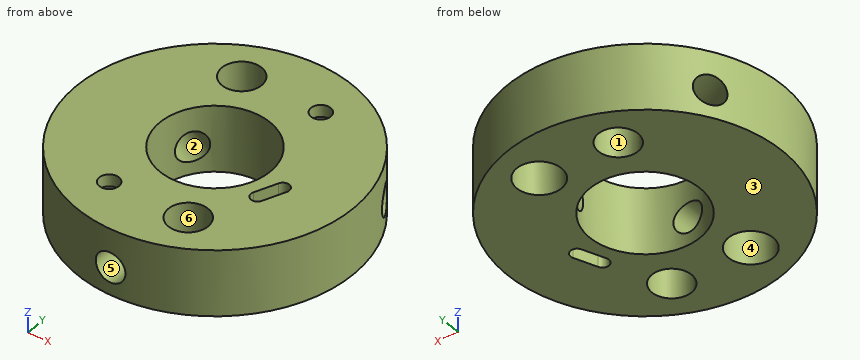
from build123d import *

# Parameters (mm, degrees)
SKETCH1_R                                      = 15.875
BOSS_EXTRUDE1_DEPTH                            = 7.62
SKETCH2_R                                      = 6.35
CUT_EXTRUDE1_DEPTH                             = 24.708556472
CIRPATTERN1_COUNT                              = 3
CBORE_FOR_2_BUTTON_HEAD_CAP_SCREW1_D           = 2.2606
CBORE_FOR_2_BUTTON_HEAD_CAP_SCREW1_CBORE_D     = 5.15874
CBORE_FOR_2_BUTTON_HEAD_CAP_SCREW1_CBORE_DEPTH = 6.2484
CIRPATTERN2_COUNT                              = 2
SKETCH42_R                                     = 2.286
CUT_EXTRUDE2_DEPTH                             = 7.62
CIRPATTERN3_COUNT                              = 2
CUT_EXTRUDE3_DEPTH                             = 24.70855664


with BuildPart() as part:
    # Sketch1 → Boss-Extrude1 (new body)
    with BuildSketch(Plane.XY):
        with Locations(Location((0, 0, 0), (0, 0, 180))):
            Circle(SKETCH1_R)
    extrude(amount=BOSS_EXTRUDE1_DEPTH)

    # Sketch2 → Cut-Extrude1 (cut, through all)
    with BuildSketch(Plane.XY.offset(7.62)):
        Circle(SKETCH2_R)
    extrude(amount=-CUT_EXTRUDE1_DEPTH, mode=Mode.SUBTRACT)

    # Sketch36 → Tap Drill for #8-32 Tap1 (revolve, cut)
    with BuildSketch(Plane(origin=(-0.450397279, -15.875, 3.175), x_dir=(0, 0, -1), z_dir=(1, 0, 0))):
        Polygon((0, 0), (0, 20.499292883), (1.7272, 19.05), (1.7272, 0), align=None)
    tap_drill_for_8_32_tap1 = revolve(axis=Axis((-0.450397279, -22.225, 3.175), (0, 1, 0)), mode=Mode.SUBTRACT)

    # CirPattern1: Tap Drill for #8-32 Tap1 ×3 about axis
    cirpattern1_axis = Axis((0, 0, 7.62), (0, 0, -1))
    for i in range(1, CIRPATTERN1_COUNT):
        add(tap_drill_for_8_32_tap1.rotate(cirpattern1_axis, i * 360 / CIRPATTERN1_COUNT), mode=Mode.SUBTRACT)

    # CBORE for #2 Button Head Cap Screw1 (through all)
    with Locations(Plane(origin=(0, 0, 0), x_dir=(-1, 0, 0), z_dir=(0, 0, -1))):
        with Locations((4.769587089, -10.050926029)):
            cbore_for_2_button_head_cap_screw1 = CounterBoreHole(CBORE_FOR_2_BUTTON_HEAD_CAP_SCREW1_D / 2, CBORE_FOR_2_BUTTON_HEAD_CAP_SCREW1_CBORE_D / 2, CBORE_FOR_2_BUTTON_HEAD_CAP_SCREW1_CBORE_DEPTH)

    # CirPattern2: CBORE for #2 Button Head Cap Screw1 ×2 about axis
    cirpattern2_axis = Axis((0, 0, 0), (0, 0, 1))
    for i in range(1, CIRPATTERN2_COUNT):
        add(cbore_for_2_button_head_cap_screw1.rotate(cirpattern2_axis, i * 360 / CIRPATTERN2_COUNT), mode=Mode.SUBTRACT)

    # Sketch42 → Cut-Extrude2 (cut)
    with BuildSketch(Plane(origin=(0, 0, 0), x_dir=(-1, 0, 0), z_dir=(0, 0, -1))):
        with Locations((4.365368762, 10.219159056)):
            Circle(SKETCH42_R)
    cut_extrude2 = extrude(amount=-CUT_EXTRUDE2_DEPTH, mode=Mode.SUBTRACT)

    # CirPattern3: Cut-Extrude2 ×2 about axis
    cirpattern3_axis = Axis((0, 0, 0), (0, 0, 1))
    for i in range(1, CIRPATTERN3_COUNT):
        add(cut_extrude2.rotate(cirpattern3_axis, i * 360 / CIRPATTERN3_COUNT), mode=Mode.SUBTRACT)

    # Sketch43 → Cut-Extrude3 (cut, through all)
    with BuildSketch(Plane(origin=(0, 0, 0), x_dir=(-1, 0, 0), z_dir=(0, 0, -1))):
        with BuildLine():
            Line((-8.025711128, -1.073137194), (-6.956985206, -3.563699487))
            ThreePointArc((-6.956985206, -3.563699487), (-7.355887027, -4.562271884), (-8.354459424, -4.163370063))
            Line((-8.354459424, -4.163370063), (-9.423185347, -1.67280777))
            ThreePointArc((-9.423185347, -1.67280777), (-9.024283525, -0.674235373), (-8.025711128, -1.073137194))
        make_face()
    extrude(amount=-CUT_EXTRUDE3_DEPTH, mode=Mode.SUBTRACT)


solid = part.part
Can you work these out from the model? Positions are in its coordinate system, mm. Face numbers are marked on the shaded views. A direction names the side the tool comes from. Give positions to 0.01 mm unless a question says otherwise; leave off trailing zeros. Loops run counter-clockwise (first coordinate to the right, second up) from the corner with the lowest first, then second, coordinate; pieces in that order, holes last. Notation, with made-up numbers: (51, 85.5) -> (79, 85.5) arc R30 cw to (79, 112.5) -> close; hole circle Ø8 at (-28, -33). An arc over 180 degrees is marked (long way). Return JSON: item names as keys, results as strings.
Q1. I want a section at A-A, the plane z = 2.5. List the corners of the cut face in (x, y) for me (3 decimals).
Checks:
{"outline": "(-14.282, 6.93) arc R15.875 ccw to (-2.04, -15.743) -> (-2.04, -6.013) arc R6.35 cw to (-5.98, 2.137) -> close; (-12.614, 9.639) -> (-4.188, 4.774) arc R6.35 cw to (4.84, 4.11) -> (13.143, 8.904) arc R15.875 ccw to start; (1.139, -15.834) arc R15.875 ccw to (14.654, 6.105) -> (6.228, 1.24) arc R6.35 cw to (1.139, -6.247) -> close; hole circle Ø5.159 at (-4.77, -10.051); hole circle Ø4.572 at (-4.365, 10.219); hole circle Ø4.572 at (4.365, -10.219); hole circle Ø5.159 at (4.77, 10.051); hole (6.957, -3.564) arc R0.76 ccw to (8.354, -4.163) -> (9.423, -1.673) arc R0.76 ccw to (8.026, -1.073) -> close"}
Q2. We'd pull the mould along Z, two halves only. Please class the marked faces 1, 2 and 3: released by +Z, released by -Z, zero draft, split by the parting line, or undercut.
Checks:
{"face 1": "zero draft", "face 2": "undercut", "face 3": "released by -Z"}
Q3. On a 3-axis mill with a long thin cutter (end or side, diameter ignored), from which of +Z, -Z, +X, -X, +Y, -Y can I reach the whole of each face in a straight line? I mean the marked faces 4, 5 and 6. Say none if no direction works.
Checks:
{"face 4": "-Z", "face 5": "-Y", "face 6": "+Z, -Z"}
Q4. I want a section at D-D, the plane z = 7. List the corners of the cut face in (x, y) for me (3 decimals), then the cut area to 3 significant figures.
Checks:
{"outline": "circle Ø31.75 at (0, 0); hole circle Ø4.572 at (-4.365, 10.219); hole circle Ø12.7 at (0, 0); hole circle Ø2.261 at (-4.77, -10.051); hole circle Ø4.572 at (4.365, -10.219); hole circle Ø2.261 at (4.77, 10.051); hole (6.957, -3.564) arc R0.76 ccw to (8.354, -4.163) -> (9.423, -1.673) arc R0.76 ccw to (8.026, -1.073) -> close", "area": "618 mm2"}
Q5. I want a section at C-C, the plane x = 3. List the corners of the cut face in (y, z) for me, then the cut area to 3 significant figures.
Checks:
{"outline": "(-15.59, 0) -> (-12.05, 0) -> (-12.05, 7.62) -> (-15.59, 7.62) -> close; (-8.39, 0) -> (-5.6, 0) -> (-5.6, 7.62) -> (-8.39, 7.62) -> close; (5.6, 0) -> (8.17, 0) -> (8.17, 6.25) -> (11.93, 6.25) -> (11.93, 0) -> (15.59, 0) -> (15.59, 7.62) -> (5.6, 7.62) -> close", "area": "101 mm2"}
Q6. For pin 1 Ø4 at (x, y) = (-4.5, -9) entering from -Z; pin 2 Ø1.5 at (y, z) = (8, 2) entering from -X; pin 3 Ø1.5 at (x, y) = (6, 11) entering from -Z; pin 4 Ø3 at (x, z) = (4, 4.5) entering from -Y, each with a flat end and sliding along its axis, tell me the tip position at first contact or that it passes through.
Checks:
{"pin 1": "stops at z = 0", "pin 2": "stops at x = -14.12", "pin 3": "stops at z = 6.25", "pin 4": "stops at y = -15.68"}
Q7. I need wall thicknesses on probe 1 along Y at (x, z) = (-3.5, 5.25); probe 2 along X at (y, z) = (-3.5, 2.25); probe 3 along X at (y, z) = (12, 4.5). Which ranges of each line are inside material? Lowest first, please.
Checks:
{"probe 1": "y = -15.48 to -12.3, -7.81 to -5.3, 5.3 to 8.1, 12.34 to 15.48", "probe 2": "x = -15.48 to -5.3, 5.3 to 6.98, 8.64 to 15.48", "probe 3": "x = -10.39 to -5.8, -2.93 to 3.08, 6.46 to 10.39"}
Q8. I want a section at B-B, the plane y = 0. List the corners of the cut face in (x, z) for me (3 decimals).
Checks:
{"outline": "(-15.875, 0) -> (-6.35, 0) -> (-6.35, 7.62) -> (-15.875, 7.62) -> close; (6.35, 0) -> (15.875, 0) -> (15.875, 7.62) -> (6.35, 7.62) -> close"}
